Geometry: final body of the model. Coordinates: model frame, mm. A direction names the side the tool comes from. Give positions to 0.01 mm unless a question says otherwise; leave off trailing zeros. Loops run counter-clockwise (first coordinate to the right, second up) from the corner with the lowest first, then second, coordinate; pieces in that order, holes last.
1. Section D-D, the plane z = 3.45. State how many separate pieces and enclosed holes the cut face has, then the cut area to 3 significant figures.
2. Section B-B, the plane x = -32. Output: boundary loops of the cut face in (y, z), then the cut area to 3 significant figures.
3. Material intervals for line 1 along Y through (x, z) = (0.5, 2.6); line 2 along Y through (x, z) = (-19.5, 4.55) (3 decimals); line 3 along X through (y, z) = (5.5, 2.8), sorted ascending.
4. Access query for faces 1 (the face through (-22.4, -8.8, 3)), 2 (the face through (-32.18, 11.33, 2.96)), 3 (the face through (22.653, -0.836, 2.958)), 4 (the face through (10.69, 20.11, 2.96)). Directions: +Z, -Z, +X, -X, +Y, -Y. A direction counts if a zero-diameter tool reaches every point of the face in a straight line with its end or side. Return the directions, or none.
5. Draft query along Y for faces 5 (the face through (-10.603, 20.036, 2.958)), 6 (the face through (-22.766, -0.796, 2.958)). Return one class per face: +Y half, -Y half, draft (parallel to the pull), parting line (faces both ways), or undercut.
6. Section A-A, the plane y = 25. Output: boundary loops of the cut face in (x, z), then the cut area to 3 significant figures.
7. First-contact query: P1, Ø1.8, axis at y = 17.5, z = 4, coming from the -X side; P2, Ø3, axis at y = -34.5, z = 3.5, coming from the -X side; P3, Ø1, axis at y = 1, z = 1.5, coming from the -X side. Flat tips, straight axial feed; report the tip coordinate or a pass-through.
8. Section C-C, the plane y = -32. Output: boundary loops of the cut face in (x, z), then the cut area to 3 significant figures.
from build123d import *

# Parameters (mm, degrees)
F0_R     = 9.45
F1_DEPTH = 6


with BuildPart() as f1:
    # F0 (on Top) → F1 (new body)
    with BuildSketch(Plane.XY):
        Polygon((11.8595659331, -15), (25.9807621135, -15), (18.9201640233, -2.7706853759), (13.302852552, 6.9587834943), (9.2066626406, 8.2897162761), (8.0631483411, 13.6695280801), (8.9614312964, 14.478345686), (7.0605980902, 17.7706853759), (0, 30), (-7.0605980902, 17.7706853759), (-12.6779095615, 8.0412165057), (-11.7824362055, 3.8283455928), (-15.8697327457, 0.1481272578), (-17.0193308171, 0.521654314), (-18.9201640233, -2.7706853759), (-25.9807621135, -15), (-11.8595659331, -15), (-0.6249429905, -15), (2.5757735649, -12.1180618689), (7.8065844046, -13.8176553379), (8.0578995207, -15), align=None)
        Circle(F0_R, mode=Mode.SUBTRACT)
        with BuildLine():
            ThreePointArc((13.4207676072, -23.3005226447), (12.0614730092, -19.25910479), (11.8595659331, -15))
            Line((11.8595659331, -15), (8.0578995207, -15))
            Line((8.0578995207, -15), (8.6399217922, -17.7381995032))
            ThreePointArc((8.6399217922, -17.7381995032), (11.3755599368, -20.2226467731), (13.4207676072, -23.3005226447))
        make_face()
        with BuildLine():
            Line((13.302852552, 6.9587834943), (18.9201640233, -2.7706853759))
            ThreePointArc((18.9201640233, -2.7706853759), (22.7096105069, -0.815989638), (26.8892283353, 0.0275356362))
            ThreePointArc((26.8892283353, 0.0275356362), (19.1613457519, 1.6397769298), (13.3222745374, 6.9524729087))
            Line((13.3222745374, 6.9524729087), (13.302852552, 6.9587834943))
        make_face()
        with BuildLine():
            ThreePointArc((15, -30), (14.5998546929, -26.5584534078), (13.4207676072, -23.3005226447))
            ThreePointArc((13.4207676072, -23.3005226447), (11.3755599368, -20.2226467731), (8.6399217922, -17.7381995032))
            Line((8.6399217922, -17.7381995032), (8.9500987041, -19.1974671419))
            Line((8.9500987041, -19.1974671419), (4.8628021639, -22.8776854769))
            Line((4.8628021639, -22.8776854769), (-0.3680086757, -21.1780920079))
            Line((-0.3680086757, -21.1780920079), (-1.5115229752, -15.7982802038))
            Line((-1.5115229752, -15.7982802038), (-0.6401191106, -15.0136646399))
            ThreePointArc((-0.6401191106, -15.0136646399), (-8.1605843982, -17.4141006567), (-13.4207676072, -23.3005226447))
            ThreePointArc((-13.4207676072, -23.3005226447), (-3.4415465922, -44.5998546929), (15, -30))
        make_face()
        Polygon((6.2786841774, -37.2124443067), (0, -40.8374443067), (-6.2786841774, -37.2124443067), (-6.2786841774, -29.9624443067), (0, -26.3374443067), (6.2786841774, -29.9624443067), align=None, mode=Mode.SUBTRACT)
        with BuildLine():
            ThreePointArc((13.3222745374, 6.9524729087), (19.1613457519, 1.6397769298), (26.8892283353, 0.0275356362))
            ThreePointArc((26.8892283353, 0.0275356362), (36.903833873, 4.7196058764), (40.9807621135, 15))
            ThreePointArc((40.9807621135, 15), (30.3002226828, 29.3646183517), (13.4684607282, 23.2729870084))
            ThreePointArc((13.4684607282, 23.2729870084), (11.8255458689, 19.9628472741), (11.041770491, 16.3514915103))
            Line((11.041770491, 16.3514915103), (12.1504448812, 17.3497464151))
            Line((12.1504448812, 17.3497464151), (17.3812557208, 15.650152946))
            Line((17.3812557208, 15.650152946), (18.5247700203, 10.270341142))
            Line((18.5247700203, 10.270341142), (14.4374734802, 6.590122807))
            Line((14.4374734802, 6.590122807), (13.3222745374, 6.9524729087))
        make_face()
        Polygon((29.0875800178, 24.0437221533), (35.3662641952, 20.4187221533), (35.3662641952, 13.1687221533), (29.0875800178, 9.5437221533), (22.8088958404, 13.1687221533), (22.8088958404, 20.4187221533), align=None, mode=Mode.SUBTRACT)
        with BuildLine():
            Line((-0.6401191106, -15.0136646399), (-0.6249429905, -15))
            Line((-0.6249429905, -15), (-11.8595659331, -15))
            ThreePointArc((-11.8595659331, -15), (-12.0614730092, -19.25910479), (-13.4207676072, -23.3005226447))
            ThreePointArc((-13.4207676072, -23.3005226447), (-8.1605843982, -17.4141006567), (-0.6401191106, -15.0136646399))
        make_face()
        with BuildLine():
            Line((7.0605980902, 17.7706853759), (8.9614312964, 14.478345686))
            Line((8.9614312964, 14.478345686), (11.041770491, 16.3514915103))
            ThreePointArc((11.041770491, 16.3514915103), (11.8255458689, 19.9628472741), (13.4684607282, 23.2729870084))
            ThreePointArc((13.4684607282, 23.2729870084), (10.6481374977, 20.0750944281), (7.0605980902, 17.7706853759))
        make_face()
        with BuildLine():
            ThreePointArc((-26.8892283353, 0.0275356362), (-22.7096105069, -0.815989638), (-18.9201640233, -2.7706853759))
            Line((-18.9201640233, -2.7706853759), (-17.0193308171, 0.521654314))
            Line((-17.0193308171, 0.521654314), (-19.6816922832, 1.3867079928))
            ThreePointArc((-19.6816922832, 1.3867079928), (-23.2011058057, 0.259799499), (-26.8892283353, 0.0275356362))
        make_face()
        with BuildLine():
            Line((-12.6779095615, 8.0412165057), (-7.0605980902, 17.7706853759))
            ThreePointArc((-7.0605980902, 17.7706853759), (-10.6481374977, 20.0750944281), (-13.4684607282, 23.2729870084))
            ThreePointArc((-13.4684607282, 23.2729870084), (-11.6161437618, 19.3194605693), (-10.9807621135, 15))
            ThreePointArc((-10.9807621135, 15), (-11.4123184715, 11.4278228138), (-12.6821554268, 8.0611917312))
            Line((-12.6821554268, 8.0611917312), (-12.6779095615, 8.0412165057))
        make_face()
        with BuildLine():
            ThreePointArc((-13.4684607282, 23.2729870084), (-38.9711431703, 22.5), (-26.8892283353, 0.0275356362))
            ThreePointArc((-26.8892283353, 0.0275356362), (-23.2011058057, 0.259799499), (-19.6816922832, 1.3867079928))
            Line((-19.6816922832, 1.3867079928), (-21.1005435853, 1.8477207269))
            Line((-21.1005435853, 1.8477207269), (-22.2440578848, 7.2275325309))
            Line((-22.2440578848, 7.2275325309), (-18.1567613447, 10.9077508659))
            Line((-18.1567613447, 10.9077508659), (-12.925950505, 9.2081573968))
            Line((-12.925950505, 9.2081573968), (-12.6821554268, 8.0611917312))
            ThreePointArc((-12.6821554268, 8.0611917312), (-11.4123184715, 11.4278228138), (-10.9807621135, 15))
            ThreePointArc((-10.9807621135, 15), (-11.6161437618, 19.3194605693), (-13.4684607282, 23.2729870084))
        make_face()
        Polygon((-35.3662641952, 13.1687221533), (-35.3662641952, 20.4187221533), (-29.0875800178, 24.0437221533), (-22.8088958404, 20.4187221533), (-22.8088958404, 13.1687221533), (-29.0875800178, 9.5437221533), align=None, mode=Mode.SUBTRACT)
    extrude(amount=F1_DEPTH)


solid = f1.part
Answers below:
1. separate pieces: 1
1. enclosed holes: 7
1. area: 2,500 mm2
2. outline: (1.26, 0) - (11.23, 0) - (11.23, 6) - (1.26, 6) - close; (22.36, 0) - (28.74, 0) - (28.74, 6) - (22.36, 6) - close
2. area: 98.0 mm2
3. line 1: y = -44.99 to -40.55, -26.63 to -21.46, -13.99 to -9.44, 9.44 to 29.13
3. line 2: y = -15 to -3.775, -2.381 to 1.328, 9.698 to 28.528
3. line 3: x = -37.59 to -21.88, -12.14 to -7.68, 7.68 to 37.59
4. face 1: +Z, -Z, -X
4. face 2: +Z, -Z
4. face 3: +Z, -Z, +X
4. face 4: +Z, -Z, +Y
5. face 5: +Y half
5. face 6: undercut
6. outline: (-37.16, 0) - (-14.8, 0) - (-14.8, 6) - (-37.16, 6) - close; (-2.89, 0) - (2.89, 0) - (2.89, 6) - (-2.89, 6) - close; (14.8, 0) - (37.16, 0) - (37.16, 6) - (14.8, 6) - close
6. area: 303 mm2
7. P1: stops at x = -40.9
7. P2: stops at x = -14.7
7. P3: stops at x = -32.52
8. outline: (-14.87, 0) - (-6.28, 0) - (-6.28, 6) - (-14.87, 6) - close; (6.28, 0) - (14.87, 0) - (14.87, 6) - (6.28, 6) - close
8. area: 103 mm2
